```python
from build123d import *

# Parameters (mm, degrees)
SKETCH1_R               = 12.7
SKETCH1_R_2             = 10.16
SKETCH1_W               = 116.84
SKETCH1_H               = 15.24
BOSS_EXTRUDE1_DEPTH     = 101.6
SKETCH2_W               = 27.184704077
SKETCH2_H               = 25.4
CUT_EXTRUDE1_DEPTH      = 6.08
CUT_EXTRUDE1_DEPTH_BACK = 21.32
SKETCH3_W               = 76.2
SKETCH3_H               = 30.48
CUT_EXTRUDE2_DEPTH      = 21.32
SKETCH4_R               = 15.24
BOSS_EXTRUDE2_DEPTH     = 30.48


with BuildPart() as part:
    # Sketch1 → Boss-Extrude1 (new body)
    with BuildSketch(Plane.XY):
        Circle(SKETCH1_R)
        Circle(SKETCH1_R_2, mode=Mode.SUBTRACT)
        with Locations((68.58, 0)):
            Rectangle(SKETCH1_W, SKETCH1_H)
    extrude(amount=BOSS_EXTRUDE1_DEPTH)

    # Sketch2 → Cut-Extrude1 (cut, two sides)
    with BuildSketch(Plane(origin=(0, 7.62, 0), x_dir=(1, 0, 0), z_dir=(0, 1, 0))) as cut_extrude1_sk:
        with Locations((0.892352039, -88.9)):
            Rectangle(SKETCH2_W, SKETCH2_H)
        with Locations((0.892352039, -12.7)):
            Rectangle(SKETCH2_W, SKETCH2_H)
    extrude(amount=CUT_EXTRUDE1_DEPTH, mode=Mode.SUBTRACT)
    extrude(cut_extrude1_sk.sketch, amount=-CUT_EXTRUDE1_DEPTH_BACK, mode=Mode.SUBTRACT)

    # Sketch3 → Cut-Extrude2 (cut, through all)
    with BuildSketch(Plane.XZ.offset(7.62)):
        with Locations((70.742352039, 50.8)):
            Rectangle(SKETCH3_W, SKETCH3_H)
    extrude(amount=-CUT_EXTRUDE2_DEPTH, mode=Mode.SUBTRACT)

    # Sketch4 → Boss-Extrude2 (add)
    with BuildSketch(Plane.XY.offset(35.56)):
        with Locations((70.742352039, 0)):
            Circle(SKETCH4_R)
    extrude(amount=BOSS_EXTRUDE2_DEPTH)


solid = part.part
```
Geometry: final body of the model. Coordinates: model frame, mm. A direction names the side the tool comes from. Coordinates: 2 decimals unless noted, no trailing zeros. Order: outer loops, then holes, each group sorted by start corner. A loop starts at its lowest first (then second) coordinate and runs counter-clockwise, first axis right, second up. Notation, with made-up numbers: (69, 22) -> (97, 22) arc R25 cw to (97, 57) -> close; hole circle Ø7 at (68.5, 17.25). An arc over 180 degrees is marked (long way). Answer in a Markdown table with one row per item.
Item 1: Ray query, L1, parallel to X at y = 0, z = 54; L2, parallel to Z at x = 40.5, y = -1; L3, parallel to Y at x = 0, z = 47. Return the intervals inside material, ascending.
Return value:
| item | result |
|---|---|
| L1 | x = -12.7 to -10.16, 10.16 to 32.64, 55.5 to 85.98, 108.84 to 127 |
| L2 | z = 0 to 35.56, 66.04 to 101.6 |
| L3 | y = -12.7 to -10.16, 10.16 to 12.7 |
Item 2: Section C-C on z = 67.5. Output: boundary loops of the cut face in (x, y).
Return value:
| item | result |
|---|---|
| outline | (10.16, -7.62) -> (127, -7.62) -> (127, 7.62) -> (10.16, 7.62) arc R12.7 ccw (long way) to start; hole circle Ø20.32 at (0, 0) |
Item 3: Section D-D on x = 94. Output: boundary loops of the cut face in (y, z), plus the area to 3 significant figures.
Return value:
| item | result |
|---|---|
| outline | (-7.62, 0) -> (7.62, 0) -> (7.62, 35.56) -> (-7.62, 35.56) -> close; (-7.62, 66.04) -> (7.62, 66.04) -> (7.62, 101.6) -> (-7.62, 101.6) -> close |
| area | 1,080 mm² |
Item 4: Section A-A on y = 0. Output: boundary loops of the cut face in (x, z), plus the area to 3 significant figures.
Return value:
| item | result |
|---|---|
| outline | (-12.7, 25.4) -> (-10.16, 25.4) -> (-10.16, 76.2) -> (-12.7, 76.2) -> close; (10.16, 25.4) -> (14.48, 25.4) -> (14.48, 0) -> (127, 0) -> (127, 101.6) -> (14.48, 101.6) -> (14.48, 76.2) -> (10.16, 76.2) -> close; hole (32.64, 35.56) -> (55.5, 35.56) -> (55.5, 66.04) -> (32.64, 66.04) -> close; hole (85.98, 35.56) -> (108.84, 35.56) -> (108.84, 66.04) -> (85.98, 66.04) -> close |
| area | 10,400 mm² |
Item 5: Access query for faces 1 (the flat face through (71, -11, 35.56)), 2 (the flat face through (71, 11, 35.56)), 3 (the flat face through (10, -3, 76.2)), 4 (the flat face through (71, 11, 66.04)). Directions: +Z, -Z, +X, -X, +Y, -Y. A direction counts if a zero-diameter tool reaches every point of the face in a straight line with its end or side. Return the directions, or none.
Return value:
| item | result |
|---|---|
| face 1 | -Z, +X, -Y |
| face 2 | -Z, +X, +Y |
| face 3 | +Z, -X, +Y, -Y |
| face 4 | +Z, +X, +Y |
Item 6: Section B-B on x = 0. Output: boundary loops of the cut face in (y, z), plus the area to 3 significant figures.
Return value:
| item | result |
|---|---|
| outline | (-12.7, 25.4) -> (-10.16, 25.4) -> (-10.16, 76.2) -> (-12.7, 76.2) -> close; (10.16, 25.4) -> (12.7, 25.4) -> (12.7, 76.2) -> (10.16, 76.2) -> close |
| area | 258 mm² |
Item 7: Draft query along Z for faces 5 (the flat face through (14.485, 0, 13)), 6 (the flat face through (45, 0, 35.56)), 7 (the flat face through (32.642, 0, 51)), 8 (the flat face through (10, -3, 25.4)). Return one class per face: released by +Z, released by -Z, zero draft, split by the parting line, or undercut.
Return value:
| item | result |
|---|---|
| face 5 | zero draft |
| face 6 | undercut |
| face 7 | undercut |
| face 8 | released by -Z |
Item 8: Contact query for flat-ended pins moving along their axis: P1, Ø8, axis at y = -2, z = 60.5, coming from the -X side; P2, Ø3, axis at x = 9, y = -10.5, coming from the -Z side; P3, Ø6, axis at x = 74.5, y = -13, coming from the +Z side; P4, Ø8.5, axis at x = 77, y = -13, coming from the -Z side. Output: stop coordinate, or through.
Return value:
| item | result |
|---|---|
| P1 | stops at x = -12.7 |
| P2 | stops at z = 25.4 |
| P3 | stops at z = 66.04 |
| P4 | stops at z = 35.56 |
